Can you work these out from the model? Positions are in its coordinate system, mm. Face numbers are marked on the shaded views. A direction names the side the tool comes from. Give positions to 0.01 mm unless a question says otherwise; leave off trailing zeros. Loops run counter-clockwise (first coordinate to the right, second up) from the corner with the lowest first, then second, coordinate; pieces in that order, holes last. Notation, with made-up numbers: (-19, -4.5) - (-1, -4.5) arc R15 ccw to (-1, 12.5) - close; hole circle Ø1 at (-11, 4). An arc over 180 degrees is marked (long way). Answer as a JSON object with one key per item and string values.
```python
from build123d import *

# Parameters (mm, degrees)
CROQUIS1_R              = 2.7
CROQUIS1_R_2            = 20
SALIENTE_EXTRUIR1_DEPTH = 6
CROQUIS2_W              = 63.14
CROQUIS2_H              = 8
SALIENTE_EXTRUIR2_DEPTH = 50
REDONDEO1_R             = 5


with BuildPart() as part:
    # Croquis1 → Saliente-Extruir1 (new body)
    with BuildSketch(Plane.XY):
        with BuildLine():
            Line((-8, -50.14), (-8, 8))
            Line((-8, 8), (55.14, 8))
            Line((55.14, 8), (55.14, -50.14))
            ThreePointArc((55.14, -50.14), (53.675533906, -53.675533906), (50.14, -55.14))
            Line((50.14, -55.14), (-3, -55.14))
            ThreePointArc((-3, -55.14), (-6.535533906, -53.675533906), (-8, -50.14))
        make_face()
        Circle(CROQUIS1_R, mode=Mode.SUBTRACT)
        with Locations((47.14, 0)):
            Circle(CROQUIS1_R, mode=Mode.SUBTRACT)
        with Locations((47.14, -47.14)):
            Circle(CROQUIS1_R, mode=Mode.SUBTRACT)
        with Locations((0, -47.14)):
            Circle(CROQUIS1_R, mode=Mode.SUBTRACT)
        with Locations((23.57, -23.57)):
            Circle(CROQUIS1_R_2, mode=Mode.SUBTRACT)
    extrude(amount=SALIENTE_EXTRUIR1_DEPTH)

    # Croquis2 → Saliente-Extruir2 (add)
    with BuildSketch(Plane(origin=(0, 0, 0), x_dir=(-1, 0, 0), z_dir=(0, 0, -1))):
        with Locations((-23.57, 12)):
            Rectangle(CROQUIS2_W, CROQUIS2_H)
    extrude(amount=-SALIENTE_EXTRUIR2_DEPTH)

    # Redondeo1
    redondeo1_edges = [part.edges().sort_by_distance(p)[0] for p in [
        (23.57, 16, 0),
    ]]
    fillet(redondeo1_edges, radius=REDONDEO1_R)


solid = part.part
```
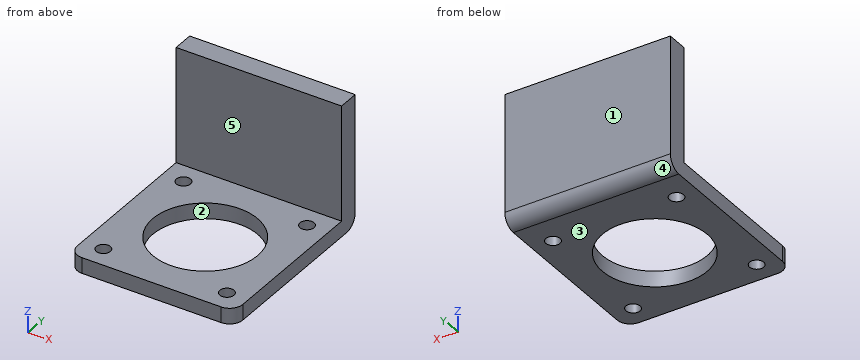
1) Imagine slicing it at B-B on y = 0. Write out the boundary of the cut face in (x, z), and give its area (3 significant figures).
Check sheet entries:
{"outline": "(-8, 0) - (-2.7, 0) - (-2.7, 6) - (-8, 6) - close; (2.7, 0) - (44.44, 0) - (44.44, 6) - (2.7, 6) - close; (49.84, 0) - (55.14, 0) - (55.14, 6) - (49.84, 6) - close", "area": "314 mm2"}
2) Which directions (+Z, -Z, +X, -X, +Y, -Y) give clear straight access to the entire face, cutting with the end or side of a thin tool? Please do the marked faces 4 and 5.
Check sheet entries:
{"face 4": "-Z, +X, -X, +Y", "face 5": "+Z, +X, -X, -Y"}
3) If we mould it in two halves opening along Y, with no side actions, what happens to the marked faces 1, 2 and 3? For each: released by +Y, released by -Y, zero draft, split by the parting line, or undercut.
Check sheet entries:
{"face 1": "released by +Y", "face 2": "undercut", "face 3": "zero draft"}
4) Imagine slicing it at A-A on y = -23.57. Write out the boundary of the cut face in (x, z), and give its area (3 significant figures).
Check sheet entries:
{"outline": "(-8, 0) - (3.57, 0) - (3.57, 6) - (-8, 6) - close; (43.57, 0) - (55.14, 0) - (55.14, 6) - (43.57, 6) - close", "area": "139 mm2"}
5) Imagine slicing it at C-C on x = 29.5. Write out the boundary of the cut face in (y, z).
Check sheet entries:
{"outline": "(-55.14, 0) - (-42.67, 0) - (-42.67, 6) - (-55.14, 6) - close; (-4.47, 0) - (11, 0) arc R5 ccw to (16, 5) - (16, 50) - (8, 50) - (8, 6) - (-4.47, 6) - close"}
6) I'm going to push flat-ended pins straight in: P1, Ø7, axis at x = 0, y = -47.14, coming from the +Z side; P2, Ø2, axis at x = 7.5, z = 12, coming from the -Y side; P3, Ø7, axis at x = 47.14, y = -47.14, coming from the -Z side. Where does each tip first touch, or does it pass through?
Check sheet entries:
{"P1": "z = 6", "P2": "y = 8", "P3": "z = 0"}
7) I need wall thicknesses on L1, parallel to X at y = -23, z = 1; L2, parallel to Y at x = 0, z = 3; L3, parallel to Y at x = 0, z = 4.35. Which ranges of each line are inside material? Lowest first, please.
Check sheet entries:
{"L1": "-8 to 3.58, 43.56 to 55.14", "L2": "-55.14 to -49.84, -44.44 to -2.7, 2.7 to 15.58", "L3": "-55.14 to -49.84, -44.44 to -2.7, 2.7 to 15.96"}
8) Imagine slicing it at D-D on z = 20.5. Write out the boundary of the cut face in (x, y), and give its area (3 significant figures).
Check sheet entries:
{"outline": "(-8, 8) - (55.14, 8) - (55.14, 16) - (-8, 16) - close", "area": "505 mm2"}
